Check sheet for the modelled part. Datum: model origin and axes. Units: mm. A direction names the side the tool comes from. Give positions to 0.01 mm unless a question says otherwise; leave off trailing zeros. Write each loop counter-clockwise with the first axis right and the second up, starting at its lowest first coordinate (ties: lowest second). Pieces come first, ordered by that corner, then holes. Notation, with made-up numbers: M 22.5,44.5 L 50.5,44.5 A23 ccw 50.5,62.5 Z; hole C -29.75,-18.75 d2. An arc over 180 degrees is marked long. Write item = value, one per line. Start each with the question number.
1) Set-up check for faces 1 (the face through (-10.549, 9.817, 3.451)), 2 (the face through (13, 0, 7)), 3 (the face through (16, -0.994, 3)), 4 (the face through (23.717, 18.096, 3.451)): record each of +Z, -Z, +X, -X, +Y, -Y from which the full face is reachable in a straight line by a thin tool's end or side.
2) Scan lines: L1, parallel to X at y = -10, z = 0.5; L2, parallel to Y at x = -6, z = 6.75; L3, parallel to X at y = -5.5, z = 3.5. Record each from-to range of solid material in increasing order.
3) Draft check along X on faces 5 (the face through (10.549, -9.817, 3.451)), 6 (the face through (25.57, 19.37, 3.45)), 7 (the face through (13, 0, 0)), 8 (the face through (16, 22.1, 3.5)). Enter one of: pulls with the +X half, pulls with the -X half, needs draft (parallel to the pull), parting line crosses it, or undercut.
4) Gauge pin test, flat ends, axial feed: pin 1 (10 mm diameter, centred on x = -1, y = 13, fed in from -Z); pin 2 (3 mm diameter, centred on x = 24, z = 2.5, fed in from -Y); pin 3 (13.5 mm diameter, centred on x = -32.02, y = 0.09, fed in from +Z) (1 decimal); pin 4 (4 mm diameter, centred on x = 3.5, z = 5, fed in from +Y). Record the tip position at first contact, or that the pin passes through.
5) Sectioned sample at B-B, the plane z = 2. Count the separate pieces of the cut face and the enclosed holes in it, then the cut area to 3 significant figures.
6) Sectioned sample at A-A, the plane x = -8.5. Record the cut outline in (y, z), then the cut area to 3 significant figures.
from build123d import *

# Parameters (mm, degrees)
F0_R     = 11.125
F0_R_2   = 12.376086
F1_DEPTH = 7


with BuildPart() as f1:
    # F0 (on Top) → F1 (new body)
    with BuildSketch(Plane.XY):
        with BuildLine():
            ThreePointArc((-17.516571, 0.089216), (-17.523634, 0.541725), (-17.544814, 0.993793))
            ThreePointArc((-17.544814, 0.993793), (-41.760355, 10.827403), (-34.318804, -14.22685))
            ThreePointArc((-34.318804, -14.22685), (-32.768784, -14.39126), (-31.210072, -14.388338))
            ThreePointArc((-31.210072, -14.388338), (-21.832298, -10.23215), (-17.551095, -0.910784))
            ThreePointArc((-17.551095, -0.910784), (-17.525205, -0.411082), (-17.516571, 0.089216))
        make_face()
        with Locations((-32.016571, 0.089216)):
            Circle(F0_R, mode=Mode.SUBTRACT)
        with BuildLine():
            ThreePointArc((14.375696, -0.993793), (14.401426, -0.497193), (14.410006, 0))
            ThreePointArc((14.410006, 0), (14.401426, 0.497193), (14.375696, 0.993793))
            ThreePointArc((14.375696, 0.993793), (10.466538, 9.904537), (1.784877, 14.299038))
            ThreePointArc((1.784877, 14.299038), (-0.255218, 14.407745), (-2.290183, 14.226852))
            ThreePointArc((-2.290183, 14.226852), (-10.640317, 9.717609), (-14.375696, 0.993793))
            ThreePointArc((-14.375696, 0.993793), (-14.409946, 0.041595), (-14.381194, -0.910784))
            ThreePointArc((-14.381194, -0.910784), (-10.146519, -10.232127), (-0.789928, -14.388338))
            ThreePointArc((-0.789928, -14.388338), (0.754468, -14.390241), (2.290198, -14.22685))
            ThreePointArc((2.290198, -14.22685), (10.640322, -9.717603), (14.375696, -0.993793))
        make_face()
        Circle(F0_R_2, mode=Mode.SUBTRACT)
        with BuildLine():
            Line((-15.511252, -24.588406), (2.290198, -14.22685))
            ThreePointArc((2.290198, -14.22685), (0.754468, -14.390241), (-0.789928, -14.388338))
            Line((-0.789928, -14.388338), (-14.490846, -22.363129))
            ThreePointArc((-14.490846, -22.363129), (-16, -22.770359), (-17.509154, -22.363129))
            Line((-17.509154, -22.363129), (-24.503051, -18.292243))
            Line((-24.503051, -18.292243), (-31.210072, -14.388338))
            ThreePointArc((-31.210072, -14.388338), (-32.768784, -14.39126), (-34.318804, -14.22685))
            Line((-34.318804, -14.22685), (-24.517354, -19.931906))
            Line((-24.517354, -19.931906), (-16.517354, -24.588406))
            ThreePointArc((-16.517354, -24.588406), (-16.014303, -24.724149), (-15.511252, -24.588406))
        make_face()
        with BuildLine():
            ThreePointArc((30.114196, 14.394545), (21.378316, 9.9726), (17.444744, 1.006207))
            ThreePointArc((17.444744, 1.006207), (17.41022, 0.006207), (17.444744, -0.993793))
            ThreePointArc((17.444744, -0.993793), (32.410518, -14.48516), (46.41022, 0.006207))
            ThreePointArc((46.41022, 0.006207), (42.997331, 9.351042), (34.36526, 14.29686))
            ThreePointArc((34.36526, 14.29686), (32.243328, 14.50238), (30.114196, 14.394545))
        make_face()
        with Locations((31.91022, 0.006207)):
            Circle(F0_R, mode=Mode.SUBTRACT)
        with BuildLine():
            ThreePointArc((14.375696, 0.993793), (14.401426, 0.497193), (14.410006, 0))
            ThreePointArc((14.410006, 0), (14.401426, -0.497193), (14.375696, -0.993793))
            Line((14.375696, -0.993793), (17.444744, -0.993793))
            ThreePointArc((17.444744, -0.993793), (17.41022, 0.006207), (17.444744, 1.006207))
            Line((17.444744, 1.006207), (14.375696, 0.993793))
        make_face()
        with BuildLine():
            ThreePointArc((-2.290183, 14.226852), (-0.255218, 14.407745), (1.784877, 14.299038))
            Line((1.784877, 14.299038), (8.491907, 18.202972))
            Line((8.491907, 18.202972), (14.48426, 21.690918))
            ThreePointArc((14.48426, 21.690918), (15.98947, 22.09815), (17.495747, 21.694885))
            Line((17.495747, 21.694885), (30.114196, 14.394545))
            ThreePointArc((30.114196, 14.394545), (32.243328, 14.50238), (34.36526, 14.29686))
            Line((34.36526, 14.29686), (16.516219, 24.591779))
            ThreePointArc((16.516219, 24.591779), (16.014611, 24.725537), (15.513537, 24.589794))
            Line((15.513537, 24.589794), (7.511249, 19.931933))
            Line((7.511249, 19.931933), (-2.290183, 14.226852))
        make_face()
        with BuildLine():
            ThreePointArc((-14.381194, -0.910784), (-14.409946, 0.041595), (-14.375696, 0.993793))
            Line((-14.375696, 0.993793), (-15.91022, 0.993793))
            Line((-15.91022, 0.993793), (-17.544814, 0.993793))
            ThreePointArc((-17.544814, 0.993793), (-17.523634, 0.541725), (-17.516571, 0.089216))
            ThreePointArc((-17.516571, 0.089216), (-17.525205, -0.411082), (-17.551095, -0.910784))
            Line((-17.551095, -0.910784), (-16.016571, -0.910784))
            Line((-16.016571, -0.910784), (-14.381194, -0.910784))
        make_face()
    extrude(amount=F1_DEPTH)


solid = f1.part
Data:
q1.face_1 = +Z, -Z, +Y
q1.face_2 = +Z, +X, -X, +Y, -Y
q1.face_3 = +Z, -Z, -Y
q1.face_4 = +Z, -Z
q2.L1 = -42.43 to -36.7, -27.33 to -21.6, -10.38 to -7.29, 7.29 to 10.38, 21.42 to 27.05, 36.77 to 42.4
q2.L2 = -19.05 to -17.42, -13.1 to -10.82, 10.82 to 13.1
q2.L3 = -45.4 to -41.64, -22.4 to -18.64, -13.32 to -11.09, 11.09 to 13.32, 18.5 to 22.24, 41.58 to 45.32
q3.face_5 = undercut
q3.face_6 = pulls with the +X half
q3.face_7 = needs draft
q3.face_8 = undercut
q4.pin_1 = 0
q4.pin_2 = -13
q4.pin_3 = through
q4.pin_4 = 18.76
q5.separate_pieces = 1
q5.enclosed_holes = 5
q5.area = 857 mm2
q6.outline = M -20.51,0 L -18.88,0 L -18.88,7 L -20.51,7 Z; M -11.64,0 L -9,0 L -9,7 L -11.64,7 Z; M 9,0 L 11.64,0 L 11.64,7 L 9,7 Z
q6.area = 48.4 mm2
